from build123d import *

# Parameters (mm, degrees)
EXTRUDE_1_DEPTH          = 10
CUT_EXTRUDE_1_DEPTH      = 74.674961826
CUT_EXTRUDE_1_DEPTH_BACK = 74.674961826
SKETCH_3_W               = 12.4
SKETCH_3_H               = 18
CUT_EXTRUDE_4_DEPTH      = 10
EXTRUDE_3_DEPTH          = 10
SKETCH_5_R               = 1.4
CUT_EXTRUDE_5_DEPTH      = 10
SKETCH_6_R               = 1.475
SKETCH_6_R_2             = 1.5
CUT_EXTRUDE_6_DEPTH      = 10
EXTRUDE_4_DEPTH          = 2
SKETCH_8_R               = 1.5
CUT_EXTRUDE_8_DEPTH      = 44.130615576
SKETCH_9_R               = 2.75
CUT_EXTRUDE_9_DEPTH      = 2
SKETCH_10_R              = 1.45
CUT_EXTRUDE_10_DEPTH     = 5


with BuildPart() as part:
    # 草图1 → 凸台-拉伸1 (new body)
    with BuildSketch(Plane(origin=(0, 0, 0), x_dir=(0, 0, -1), z_dir=(1, 0, 0))):
        with BuildLine():
            Line((-32.097226847, 5.621533559), (-15, 12))
            Line((-15, 12), (15, 12))
            Line((15, 12), (32.097226847, 5.621533559))
            ThreePointArc((32.097226847, 5.621533559), (36, 0), (32.097226847, -5.621533559))
            Line((32.097226847, -5.621533559), (15, -12))
            Line((15, -12), (-15, -12))
            Line((-15, -12), (-32.097226847, -5.621533559))
            ThreePointArc((-32.097226847, -5.621533559), (-36, 0), (-32.097226847, 5.621533559))
        make_face()
    extrude(amount=EXTRUDE_1_DEPTH)

    # 草图2 → 切除-拉伸1 (cut, two sides: drawn at the far end of the back side and taken through both)
    with BuildSketch(Plane.XY.offset(36).offset(-CUT_EXTRUDE_1_DEPTH_BACK)):
        Polygon((0, -3.5), (3, -3.5), (3, -6), (7, -6), (7, 6), (3, 6), (3, 3.5), (0, 3.5), align=None)
    extrude(amount=CUT_EXTRUDE_1_DEPTH + CUT_EXTRUDE_1_DEPTH_BACK, mode=Mode.SUBTRACT)

    # 草图3 → 切除-拉伸4 (cut)
    with BuildSketch(Plane(origin=(10, 0, 0), x_dir=(0, 0, -1), z_dir=(1, 0, 0))):
        with Locations((0, 3)):
            Rectangle(SKETCH_3_W, SKETCH_3_H)
    extrude(amount=-CUT_EXTRUDE_4_DEPTH, mode=Mode.SUBTRACT)

    # 草图4 → 凸台-拉伸3 (add)
    with BuildSketch(Plane(origin=(10, 0, 0), x_dir=(0, 0, -1), z_dir=(1, 0, 0))):
        Polygon((-6.2, 17.5), (6.2, 17.5), (6.2, 12), (9.2, 12), (9.2, 20.5), (-9.2, 20.5), (-9.2, 12), (-6.2, 12), align=None)
    extrude(amount=-EXTRUDE_3_DEPTH)

    # 草图5 → 切除-拉伸5 (cut)
    with BuildSketch(Plane(origin=(10, 0, 0), x_dir=(0, 0, -1), z_dir=(1, 0, 0))):
        with Locations((0, -8.5)):
            Circle(SKETCH_5_R)
        with Locations((0, 20)):
            Circle(SKETCH_5_R)
    extrude(amount=-CUT_EXTRUDE_5_DEPTH, mode=Mode.SUBTRACT)

    # 草图6 → 切除-拉伸6 (cut)
    with BuildSketch(Plane(origin=(10, 0, 0), x_dir=(0, 0, -1), z_dir=(1, 0, 0))):
        with Locations((0, 20)):
            Circle(SKETCH_6_R)
        with Locations((0, -8.5)):
            Circle(SKETCH_6_R_2)
    extrude(amount=-CUT_EXTRUDE_6_DEPTH, mode=Mode.SUBTRACT)

    # 草图7 → 凸台-拉伸4 (add)
    with BuildSketch(Plane(origin=(10, 0, 0), x_dir=(0, 0, -1), z_dir=(1, 0, 0))):
        Polygon((8.2, -10), (20.360920843, -10), (21.2, -9.686964542), (21.2, 9.686964542), (20.360920843, 10), (8.2, 10), align=None)
    extrude(amount=EXTRUDE_4_DEPTH)

    # 草图8 → 切除-拉伸8 (cut, through all)
    with BuildSketch(Plane(origin=(12, 0, 0), x_dir=(0, 0, -1), z_dir=(1, 0, 0))):
        with Locations((11.7, 0)):
            Circle(SKETCH_8_R)
        with Locations((17.7, 0)):
            Circle(SKETCH_8_R)
    extrude(amount=-CUT_EXTRUDE_8_DEPTH, mode=Mode.SUBTRACT)

    # 草图9 → 切除-拉伸9 (cut)
    with BuildSketch(Plane.ZY.offset(-7)):
        with Locations(Location((-17.7, 0, 0), (0, 0, 270))):
            Circle(SKETCH_9_R)
        with Locations(Location((-11.7, 0, 0), (0, 0, 270))):
            Circle(SKETCH_9_R)
    extrude(amount=-CUT_EXTRUDE_9_DEPTH, mode=Mode.SUBTRACT)

    # 草图10 → 切除-拉伸10 (cut)
    with BuildSketch(Plane(origin=(12, 0, 0), x_dir=(0, 0, -1), z_dir=(1, 0, 0))):
        with Locations((11.2, 8)):
            Circle(SKETCH_10_R)
        with Locations((11.2, -8)):
            Circle(SKETCH_10_R)
    extrude(amount=-CUT_EXTRUDE_10_DEPTH, mode=Mode.SUBTRACT)


solid = part.part
Can you work these out from the model? Positions are in its coordinate system, mm. A direction names the side the tool comes from. Coordinates: 2 decimals unless noted, no trailing zeros. Write each loop counter-clockwise with the first axis right and the second up, starting at its lowest first coordinate (ties: lowest second). Pieces come first, ordered by that corner, then holes. Notation, with made-up numbers: (-31.75, 82) - (18.25, 82) arc R10 cw to (18.25, 88) - close; hole circle Ø9 at (5.25, 53). An arc over 180 degrees is marked (long way). Return JSON: item names as keys, results as strings. Group by question number.
Item 1: I'm going to push flat-ended pins straight in: pin 1 Ø1 at (x, z) = (11.5, -15.5) entering from -Y; pin 2 Ø0.8 at (x, y) = (1.5, -4.5) entering from +Z; pin 3 Ø4 at (x, y) = (6, 17) entering from -Z. Where does each tip first touch, or does it pass through?
Item 2: If we section it at C-C (x = 8): Write out the boundary of the cut face in (y, z) (3 decimals).
Item 3: If we section it at D-D (y = 0): Write out the boundary of the cut face in (x, z), then the cut area to 3 significant figures.
Item 4: If we section it at A-A (x = 2.25): Write out the boundary of the cut face in (y, z) (3 decimals).
Item 5: Please list where these lines run through material, in increasing order: probe 1 along Y at (x, z) = (5.75, -0.5); probe 2 along Z at (x, y) = (8, -1.5); probe 3 along Y at (x, z) = (3.25, 8.5).
Item 6: We'd pull the mould along X, two halves only. Please class faces 1 (the face through (5.07, 18.526, 0.04)), 2 (the face through (0, 10, 8)), 3 (the face through (7, 0, 21)): pulls with the +X half, pulls with the -X half, needs draft (parallel to the pull), parting line crosses it, or undercut.
Item 7: Which directions (+Z, -Z, +X, -X, +Y, -Y) give clear straight access to the entire face, cutting with the end or side of a thin tool? Please do faces 4 (the face through (6, 9, -6.2)), 5 (the face through (5, 6, 18)), 6 (the face through (11, 10, -14)), 7 (the face through (11, 0, -21.2)).
Item 8: If we section it at B-B (z = -4): Write out the boundary of the cut face in (x, y), then the cut area to 3 significant figures.
Return value:
{
 "1": {"pin 1": "stops at y = -10", "pin 2": "stops at z = 34.38", "pin 3": "stops at z = -9.2"},
 "2": {"outline": "(-12, -15) - (-5.622, -32.097) arc R6 ccw to (5.622, -32.097) - (12, -15) - (12, -9.2) - (20.5, -9.2) - (20.5, -1.388) arc R1.475 cw (long way) to (20.5, 1.388) - (20.5, 9.2) - (12, 9.2) - (12, 15) - (5.622, 32.097) arc R6 ccw to (-5.622, 32.097) - (-12, 15) - close; hole circle Ø3 at (-8.5, 0); hole circle Ø2.9 at (-8, -11.2); hole (-6, -6.2) - (17.5, -6.2) - (17.5, 6.2) - (-6, 6.2) - close; hole circle Ø5.5 at (0, -17.7); hole circle Ø5.5 at (0, -11.7); hole circle Ø2.9 at (8, -11.2)"},
 "3": {"outline": "(7, -36) - (10, -36) - (10, -21.2) - (12, -21.2) - (12, -19.2) - (9, -19.2) - (9, -20.45) - (7, -20.45) - close; (7, -14.95) - (9, -14.95) - (9, -16.2) - (12, -16.2) - (12, -13.2) - (9, -13.2) - (9, -14.45) - (7, -14.45) - close; (7, -8.95) - (9, -8.95) - (9, -10.2) - (12, -10.2) - (12, -8.2) - (10, -8.2) - (10, -6.2) - (7, -6.2) - close; (7, 6.2) - (10, 6.2) - (10, 36) - (7, 36) - close", "area": "165 mm^2"},
 "4": {"outline": "(-12, -15) - (-5.622, -32.097) arc R6 ccw to (-3.5, -34.873) - (-3.5, -6.2) - (-6, -6.2) - (-6, 6.2) - (-3.5, 6.2) - (-3.5, 34.873) arc R6 ccw to (-5.622, 32.097) - (-12, 15) - close; (3.5, -34.873) arc R6 ccw to (5.622, -32.097) - (12, -15) - (12, -9.2) - (20.5, -9.2) - (20.5, -1.388) arc R1.475 cw (long way) to (20.5, 1.388) - (20.5, 9.2) - (12, 9.2) - (12, 15) - (5.622, 32.097) arc R6 ccw to (3.5, 34.873) - (3.5, 6.2) - (17.5, 6.2) - (17.5, -6.2) - (3.5, -6.2) - close; hole circle Ø3 at (-8.5, 0)"},
 "5": {"probe 1": "y = -12 to -9.91, -7.09 to -6, 17.5 to 18.61", "probe 2": "z = -35.81 to -20, -15.4 to -14, -9.4 to -6.2, 6.2 to 35.81", "probe 3": "y = -12 to -6, 6 to 20.5"},
 "6": {"face 1": "needs draft", "face 2": "pulls with the -X half", "face 3": "undercut"},
 "7": {"face 4": "+X, -X", "face 5": "+Z, -Z", "face 6": "+Z, -Z, +X, +Y", "face 7": "-Z, +X, +Y, -Y"},
 "8": {"outline": "(0, -12) - (10, -12) - (10, -6) - (0, -6) - close; (0, 17.5) - (10, 17.5) - (10, 20.5) - (0, 20.5) - close", "area": "90.0 mm^2"}
}
